Verification items for the finished model (mm, model axes). Face numbers are marked on the shaded views. Round coordinates to 2 decimals unless told otherwise and drop trailing zeros. Write each loop counter-clockwise with the first axis right and the second up, starting at its lowest first coordinate (ties: lowest second). Pieces come first, ordered by that corner, then holes. Notation, with made-up numbers: M -38.75,81 L -24.75,81 A16 ccw -24.75,105 Z; hole C 48.25,-23 d1. An arc over 180 degrees is marked long. Answer in a Markdown table with one row per item. Add a question column.
1. Sectioned sample at B-B on z = 17.5. Record the cut outline in (x, y).
2. Go/stop test with flat-tipped pins: pin 1 Ø8 at (y, z) = (62, 11.5) entering from -X; pin 2 Ø5 at (y, z) = (73, 28.5) entering from -X. Record where each tip stops, or that it passes through.
3. Sectioned sample at D-D on x = -12.75. Count the separate pieces of the cut face and the enclosed holes in it, plus the area to 3 significant figures.
4. Material ranges on probe 1 along Y at (x, z) = (-10.75, 21); probe 2 along Y at (x, z) = (-15.75, 18); probe 3 along X at (y, z) = (21.5, 13.5), recorded low to high.
5. Sectioned sample at A-A on y = 28.5. Record the cut outline in (x, z).
6. Draft check along Z on the marked faces 1, 2, 3 and 4. Enter one of: pulls with the +Z half, pulls with the -Z half, needs draft (parallel to the pull), parting line crosses it, or undercut.
7. Sectioned sample at C-C on z = 4. Record the cut outline in (x, y).
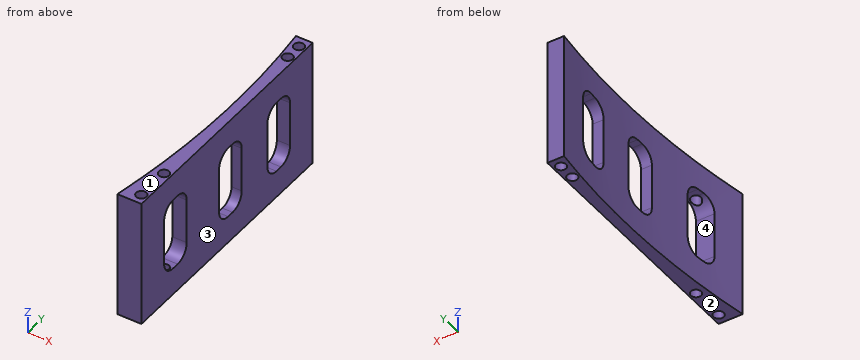
```python
from build123d import *

# Parameters (mm, degrees)
RESSALTO_EXTRUS_O1_DEPTH = 37.2
FILETE3_R                = 10
FILETE4_R                = 10
ESBO_O3_W                = 64.493903811
ESBO_O3_H                = 22.028162523
CORTE_EXTRUS_O2_DEPTH    = 126.622328301
ESBO_O4_W                = 55.088928671
ESBO_O4_H                = 123.119514717
CORTE_EXTRUS_O3_DEPTH    = 126.622328159
ESBO_O5_W                = 12.155718474
ESBO_O5_H                = 25
CORTE_EXTRUS_O4_DEPTH    = 120.46824597
CORTE_EXTRUS_O5_DEPTH    = 96.020543125
ESBO_O7_R                = 1.5
CORTE_EXTRUS_O6_DEPTH    = 97.384450815


with BuildPart() as part:
    # Esboço1 → Ressalto-extrusão1 (new body)
    with BuildSketch(Plane.XY):
        with BuildLine():
            ThreePointArc((-10, 0), (0, -10), (10, 0))
            Line((10, 0), (20, 0))
            ThreePointArc((20, 0), (14.071698091, 40.495175194), (14.829943665, 81.414963086))
            ThreePointArc((14.829943665, 81.414963086), (11.193742071, 116.066691762), (-16.576524471, 95.024435265))
            Line((-16.576524471, 95.024435265), (-16.487894969, 94.437265709))
            Line((-16.487894969, 94.437265709), (-16.369382775, 93.652123615))
            ThreePointArc((-16.369382775, 93.652123615), (-13.756795166, 46.654405302), (-20, 0))
            Line((-20, 0), (-10, 0))
        make_face()
    extrude(amount=RESSALTO_EXTRUS_O1_DEPTH)

    # Filete3
    # the kernel refuses this fillet: 10 mm, written as the material it takes off along each edge
    with BuildSketch(Plane(origin=(20, 0, -29.463728433), x_dir=(-0.20232831186330175, 0.9793177493635794, 0), z_dir=(0, 0, 1))) as filete3_piece_1:
        with BuildLine():
            CenterArc((12.021201201, 9.997221658), FILETE3_R, 181.169168083, 87.480189)
            Line((2.023283119, 9.793177494), (1.823324757, 9.78909661))
            ThreePointArc((1.823324757, 9.78909661), (0.815778009, 4.937054409), (-0.19586355, 0.040465662))
            Line((-0.19586355, 0.040465662), (0.004714197, -0.199944433))
            ThreePointArc((0.004714197, -0.199944433), (5.892745687, -0.130541448), (11.780777177, -0.199944433))
            Line((11.780777177, -0.199944433), (11.785491373, 0))
        make_face()
    extrude(amount=96.127456867, mode=Mode.SUBTRACT)
    with BuildSketch(Plane(origin=(-20, 0, -29.463728433), x_dir=(1, 0, 0), z_dir=(0, 0, 1))) as filete3_piece_2:
        with BuildLine():
            CenterArc((12.222685959, 9.749854723), FILETE3_R, 169.67749742, 87.480189)
            Line((2.384538574, 11.541740887), (2.187775626, 11.57757861))
            ThreePointArc((2.187775626, 11.57757861), (1.06442773, 5.797282674), (-0.194855317, 0.045071116))
            Line((-0.194855317, 0.045071116), (0, -0.2))
            ThreePointArc((0, -0.2), (5, -0.2), (9.955546281, -0.194997094))
            Line((9.955546281, -0.194997094), (10, 0))
        make_face()
    extrude(amount=96.127456867, mode=Mode.SUBTRACT)

    # Filete4
    filete4_edges = [part.edges().sort_by_distance(p)[0] for p in [
        (10, 0, 18.6),
        (-10, 0, 18.6),
    ]]
    fillet(filete4_edges, radius=FILETE4_R)

    # Esboço3 → Corte-extrusão2 (cut, through all)
    with BuildSketch(Plane.XY.offset(37.2)):
        with Locations((-2.119172362, 0.527659626)):
            Rectangle(ESBO_O3_W, ESBO_O3_H)
    extrude(amount=-CORTE_EXTRUS_O2_DEPTH, mode=Mode.SUBTRACT)

    # Esboço4 → Corte-extrusão3 (cut, through all)
    with BuildSketch(Plane.XY.offset(37.2)):
        with Locations((16.946535692, 73.101498246)):
            Rectangle(ESBO_O4_W, ESBO_O4_H)
    extrude(amount=-CORTE_EXTRUS_O3_DEPTH, mode=Mode.SUBTRACT)

    # Esboço5 → Corte-extrusão4 (cut, through all)
    with BuildSketch(Plane.XY.offset(37.2)):
        with Locations((-16.675787881, 99.653989291)):
            Rectangle(ESBO_O5_W, ESBO_O5_H)
    extrude(amount=-CORTE_EXTRUS_O4_DEPTH, mode=Mode.SUBTRACT)

    # Esboço6 → Corte-extrusão5 (cut, through all)
    with BuildSketch(Plane(origin=(-10.597928644, 0, 0), x_dir=(0, 0, -1), z_dir=(1, 0, 0))):
        with BuildLine():
            Line((-25.2, 77.153989291), (-12, 77.153989291))
            ThreePointArc((-12, 77.153989291), (-9.171572875, 75.982416416), (-8, 73.153989291))
            Line((-8, 73.153989291), (-8, 71.153989291))
            ThreePointArc((-8, 71.153989291), (-9.171572875, 68.325562166), (-12, 67.153989291))
            Line((-12, 67.153989291), (-25.2, 67.153989291))
            ThreePointArc((-25.2, 67.153989291), (-28.028427125, 68.325562166), (-29.2, 71.153989291))
            Line((-29.2, 71.153989291), (-29.2, 73.153989291))
            ThreePointArc((-29.2, 73.153989291), (-28.028427125, 75.982416416), (-25.2, 77.153989291))
        make_face()
        with BuildLine():
            Line((-25.2, 55.831740887), (-12, 55.831740887))
            ThreePointArc((-12, 55.831740887), (-9.171572875, 54.660168012), (-8, 51.831740887))
            Line((-8, 51.831740887), (-8, 49.831740887))
            ThreePointArc((-8, 49.831740887), (-9.171572875, 47.003313762), (-12, 45.831740887))
            Line((-12, 45.831740887), (-25.2, 45.831740887))
            ThreePointArc((-25.2, 45.831740887), (-28.028427125, 47.003313762), (-29.2, 49.831740887))
            Line((-29.2, 49.831740887), (-29.2, 51.831740887))
            ThreePointArc((-29.2, 51.831740887), (-28.028427125, 54.660168012), (-25.2, 55.831740887))
        make_face()
        with BuildLine():
            Line((-25.2, 31.541740887), (-12, 31.541740887))
            ThreePointArc((-12, 31.541740887), (-9.171572875, 30.370168012), (-8, 27.541740887))
            Line((-8, 27.541740887), (-8, 25.541740887))
            ThreePointArc((-8, 25.541740887), (-9.171572875, 22.713313762), (-12, 21.541740887))
            Line((-12, 21.541740887), (-25.2, 21.541740887))
            ThreePointArc((-25.2, 21.541740887), (-28.028427125, 22.713313762), (-29.2, 25.541740887))
            Line((-29.2, 25.541740887), (-29.2, 27.541740887))
            ThreePointArc((-29.2, 27.541740887), (-28.028427125, 30.370168012), (-25.2, 31.541740887))
        make_face()
    extrude(amount=-CORTE_EXTRUS_O5_DEPTH, mode=Mode.SUBTRACT)

    # Esboço7 → Corte-extrusão6 (cut, through all)
    with BuildSketch(Plane.XY.offset(37.2)):
        with Locations((-12.597928644, 14.541740887)):
            Circle(ESBO_O7_R)
        with Locations((-12.597928644, 84.153989291)):
            Circle(ESBO_O7_R)
        with Locations((-12.597928644, 79.153989291)):
            Circle(ESBO_O7_R)
        with Locations((-12.597928644, 24.541740887)):
            Circle(ESBO_O7_R)
    extrude(amount=-CORTE_EXTRUS_O6_DEPTH, mode=Mode.SUBTRACT)


solid = part.part
```
Geometry check:
| question | item | result |
|---|---|---|
| 1 | outline | M -17.62,11.54 L -10.6,11.54 L -10.6,21.54 L -16,21.54 A250 cw Z; M -15.48,87.15 A250 cw -14.44,77.15 L -10.6,77.15 L -10.6,87.15 Z; M -14.8,31.54 L -10.6,31.54 L -10.6,45.83 L -13.79,45.83 A250 cw Z; M -13.8,67.15 A250 cw -13.57,55.83 L -10.6,55.83 L -10.6,67.15 Z; hole C -12.6,14.54 d3; hole C -12.6,79.15 d3; hole C -12.6,84.15 d3 |
| 2 | pin 1 | stops at x = -13.76 |
| 2 | pin 2 | stops at x = -14.3 |
| 3 | separate pieces | 5 |
| 3 | enclosed holes | 2 |
| 3 | area | 1,840 mm2 |
| 4 | probe 1 | y = 11.54 to 21.54, 31.54 to 45.83, 55.83 to 67.15, 77.15 to 87.15 |
| 4 | probe 2 | y = 11.54 to 21.54 |
| 4 | probe 3 | x = -16.01 to -10.6 |
| 5 | outline | M -15.12,0 L -10.6,0 L -10.6,8.12 L -15.12,8.12 Z; M -15.12,29.08 L -10.6,29.08 L -10.6,37.2 L -15.12,37.2 Z |
| 6 | face 1 | pulls with the +Z half |
| 6 | face 2 | pulls with the -Z half |
| 6 | face 3 | needs draft |
| 6 | face 4 | undercut |
| 7 | outline | M -17.62,11.54 L -10.6,11.54 L -10.6,87.15 L -15.48,87.15 A250 cw Z; hole C -12.6,14.54 d3; hole C -12.6,24.54 d3; hole C -12.6,79.15 d3; hole C -12.6,84.15 d3 |
